Part model, mm, in its own coordinate system. A direction names the side the tool comes from. Coordinates: 2 decimals unless noted, no trailing zeros. Loops run counter-clockwise (first coordinate to the right, second up) from the corner with the lowest first, then second, coordinate; pieces in that order, holes last. Notation, with made-up numbers: (28.25, -30.5) -> (51.25, -30.5) arc R10 cw to (51.25, -11.5) -> close; hole circle Ø5 at (-30, 41). An arc over 180 degrees is marked (long way). Use one line per item in the form item = value. Start each with the question number.
(1) Band-saw the part on B-B on y = 7.25. Give the cut face in (x, z).
(2) Band-saw the part on A-A on z = 0. Give the cut face in (x, y), then the cut area to 3 significant figures.
(3) 3-axis set-ups, long thin cutter, end or side, ignore diameter. For faces 1 (the flat face through (-3, 4, 28)), 2 (the cylindrical face through (-26.253, 6.958, -0.121)): which of +Z, -Z, +X, -X, +Y, -Y reach the whole face in a straight line?
(4) Band-saw the part on C-C on z = -29. Give the cut face in (x, y), then the cut area to 3 significant figures.
(5) Drill centre lines: L1, parallel to Z at x = 0, y = 7.5; L2, parallel to Z at x = -3, y = 2.75; L3, parallel to Y at x = -30, z = -3. Where is each one in solid material? Low to high. Write a range as [from, to].
(6) Mould opens along X. For faces 3 (the flat face through (-4, 2, -29)), 4 (the flat face through (-34.5, 5, 0)) say: +X half, -X half, draft (parallel to the pull), parting line (faces both ways), or undercut.
(7) Pin check, flat tips, straight feed: P1, Ø1, axis at x = 13.5, z = -27.5, coming from the -Y side; P2, Ø2, axis at x = -26, y = 6.5, coming from the -Z side; P3, Ø4.5, axis at y = 1.5, z = -29.5, coming from the +X side; P4, Ø1.2, axis at y = 2, z = 30, coming from the -X side. Stop position of each tip, or through.
(8) Band-saw the part on D-D on x = 21. Give the cut face in (y, z), then the cut area to 3 significant figures.
Autodesk Inventor part; units mm, degrees
ref_plane "YZ Plane" through (0, 0, 0) normal (1, 0, 0) x (0, 1, 0)
ref_plane "XZ Plane" through (0, 0, 0) normal (0, 1, 0) x (-1, 0, 0)
ref_plane "XY Plane" through (0, 0, 0) normal (0, 0, 1) x (1, 0, 0)
sketch "Sketch1" plane through (0, 0, 0) normal (0, 1, 0) x (-1, 0, 0)
  circle A0 centre (0, 0) radius 39.5
  circle A1 centre (0, 0) radius 10
  circle A2 centre (0, 0) radius 29
  circle A3 centre (29, 0) radius 2.75
  circle A4 centre (0, 29) radius 2.75
  circle A5 centre (-29, 0) radius 2.75
  circle A6 centre (0, -29) radius 2.75
  dimension "d2" = 58
  dimension "d0" = 79
  dimension "d1" = 20
  dimension "d3" = 5.5
  dimension "d6" = 360
extrude "Extrusion1" add sketch "Sketch1" along normal blind 10 contours A0 | A3 A2 A6 A5 A4
sketch "Sketch2" plane through (0, 0, 0) normal (0, -1, 0) x (1, 0, 0)
  circle A0 centre (0, -29) radius 2.75
  circle A1 centre (0, 0) radius 29
  circle A2 centre (29, 0) radius 2.75
  circle A3 centre (29, 0) radius 4
  circle A4 centre (0, 29) radius 4
  circle A5 centre (-29, 0) radius 4
  circle A6 centre (0, -29) radius 4
  line L0 (25, 2.3094) -> (29, 4.6188)
  line L1 (29, 4.6188) -> (33, 2.3094)
  line L2 (33, 2.3094) -> (33, -2.3094)
  line L3 (33, -2.3094) -> (29, -4.6188)
  line L4 (29, -4.6188) -> (25, -2.3094)
  line L5 (25, -2.3094) -> (25, 2.3094)
  line L6 (-4, -26.6906) -> (0, -24.3812)
  line L7 (0, -24.3812) -> (4, -26.6906)
  line L8 (4, -26.6906) -> (4, -31.3094)
  line L9 (4, -31.3094) -> (0, -33.6188)
  line L10 (0, -33.6188) -> (-4, -31.3094)
  line L11 (-4, -31.3094) -> (-4, -26.6906)
  line L12 (-33, 2.3094) -> (-29, 4.6188)
  line L13 (-29, 4.6188) -> (-25, 2.3094)
  line L14 (-25, 2.3094) -> (-25, -2.3094)
  line L15 (-25, -2.3094) -> (-29, -4.6188)
  line L16 (-29, -4.6188) -> (-33, -2.3094)
  line L17 (-33, -2.3094) -> (-33, 2.3094)
  line L18 (-4, 31.3094) -> (0, 33.6188)
  line L19 (0, 33.6188) -> (4, 31.3094)
  line L20 (4, 31.3094) -> (4, 26.6906)
  line L21 (4, 26.6906) -> (0, 24.3812)
  line L22 (0, 24.3812) -> (-4, 26.6906)
  line L23 (-4, 26.6906) -> (-4, 31.3094)
  circle A7 centre (0, 29) radius 2.75
  circle A8 centre (-29, 0) radius 2.75
  point P0 (25, 0)
  point P1 (-4, -29)
  point P2 (-33, 0)
  point P3 (-4, 29)
  dimension "d10" = 8
  dimension "d13" = 360
extrude "Extrusion2" cut sketch "Sketch2" against normal blind 4 contours A0 A1 A6 | A0 A1 A6 | A6 L7 L8 A1 | A1 L8 A6 | A6 L11 A1 | A1 L11 L6 A6 | L8 L9 A6 | A6 L6 L7 | A6 L10 L11 | L4 A3 A1 | A1 A3 L3 L4 | L9 L10 A6 | L15 L16 A5 A1 | A1 A5 L15 | A3 A1 A2 | A1 A2 A3 | L4 L5 A3 | A5 A1 A8 | A1 A8 A5 | A5 L14 L15 | A3 L2 L3 | L5 L0 A3 | L16 L17 A5 | A5 L13 L14 | A3 L1 L2 | L0 A1 A3 | L17 L12 A5 | A5 A1 L13 | A1 L0 L1 A3 | A5 L12 L13 A1 | L20 L21 A4 A1 | A1 A4 L20 | L23 A4 A1 | A1 A4 L22 L23 | A4 A1 A7 | A1 A7 A4 | A4 L19 L20 | L23 L18 A4 | L21 L22 A4 | A4 L18 L19
sketch "Sketch3" plane through (0, 10, 0) normal (0, 1, 0) x (1, 0, 0)
  line L0 (-34.5, 50.157) -> (-34.5, -49.8555)
  circle A0 centre (0, 0) radius 39.5
  point P0 (-34.5, -19.2354)
  point P1 (-34.5, 19.2354)
  dimension "d18" = 5
extrude "Extrusion3" cut sketch "Sketch3" along normal through all both and the other way through all contours L0 A0 picked at (-35.5583, 3.956)
properties part number "Adapter Plate"
A:
q1.outline = (-34.5, -19.24) arc R39.5 ccw (long way) to (-34.5, 19.24) -> close; hole circle Ø5.5 at (-29, 0); hole circle Ø20 at (0, 0); hole circle Ø5.5 at (0, -29); hole circle Ø5.5 at (0, 29); hole circle Ø5.5 at (29, 0)
q2.outline = (-34.5, 0) -> (-33, 0) -> (-33, 4) -> (-31.75, 4) -> (-31.75, 10) -> (-34.5, 10) -> close; (-26.25, 4) -> (-25, 4) -> (-25, 0) -> (-10, 0) -> (-10, 10) -> (-26.25, 10) -> close; (10, 0) -> (25, 0) -> (25, 4) -> (26.25, 4) -> (26.25, 10) -> (10, 10) -> close; (31.75, 4) -> (33, 4) -> (33, 0) -> (39.5, 0) -> (39.5, 10) -> (31.75, 10) -> close
q2.area = 410 mm²
q3.face_1 = -Y
q3.face_2 = +Y, -Y
q4.outline = (-26.82, 0) -> (-4, 0) -> (-4, 4) -> (-2.75, 4) -> (-2.75, 10) -> (-26.82, 10) -> close; (2.75, 4) -> (4, 4) -> (4, 0) -> (26.82, 0) -> (26.82, 10) -> (2.75, 10) -> close
q4.area = 471 mm²
q5.L1 = [-39.5, -31.75], [-26.25, -10], [10, 26.25], [31.75, 39.5]
q5.L2 = [-39.39, -31.89], [-26.11, -9.54], [9.54, 26.11], [31.89, 39.39]
q5.L3 = [4, 10]
q6.face_3 = undercut
q6.face_4 = -X half
q7.P1 = 0
q7.P2 = -30.58
q7.P3 = 28.6
q7.P4 = -26.38
q8.outline = (0, -33.46) -> (10, -33.46) -> (10, 33.46) -> (0, 33.46) -> close
q8.area = 669 mm²
